```python
from build123d import *

# Parameters (mm, degrees)
SKETCH3_W           = 59
SKETCH3_H           = 36
SKETCH3_W_2         = 44
SKETCH3_H_2         = 21
BOSS_EXTRUDE1_DEPTH = 10
SKETCH3_2_W         = 59
SKETCH3_2_H         = 36
SKETCH3_2_W_2       = 44
SKETCH3_2_H_2       = 21
BOSS_EXTRUDE2_DEPTH = 5
SKETCH4_W           = 23.855112314
SKETCH4_H           = 12
BOSS_EXTRUDE3_DEPTH = 36.6
REVOLVE1_ANGLE      = 20
BOSS_EXTRUDE4_DEPTH = 10
BOSS_EXTRUDE5_REACH = 83.498
SKETCH9_W           = 12
SKETCH9_H           = 10.265164511
SKETCH3_4_W         = 59
SKETCH3_4_H         = 36
SKETCH3_4_W_2       = 44
SKETCH3_4_H_2       = 21
BOSS_EXTRUDE6_DEPTH = 7.65
BOSS_EXTRUDE7_START = 7.65
SKETCH3_5_W         = 59
SKETCH3_5_H         = 36
SKETCH3_5_W_2       = 44
SKETCH3_5_H_2       = 21
BOSS_EXTRUDE7_DEPTH = 25


with BuildPart() as part:
    # Sketch3 → Boss-Extrude1 (new body)
    with BuildSketch(Plane.XY):
        Rectangle(SKETCH3_W, SKETCH3_H)
        Rectangle(SKETCH3_W_2, SKETCH3_H_2, mode=Mode.SUBTRACT)
    extrude(amount=BOSS_EXTRUDE1_DEPTH)

    # Sketch3<2> → Boss-Extrude2 (add)
    # profile 1 of 2: a face of its own
    with BuildSketch(Plane.XY):
        Rectangle(SKETCH3_2_W, SKETCH3_2_H)
        Rectangle(SKETCH3_2_W_2, SKETCH3_2_H_2, mode=Mode.SUBTRACT)
    # profile 2 of 2: a face of its own
    with BuildSketch(Plane.XY):
        Rectangle(SKETCH3_2_W_2, SKETCH3_2_H_2)
    extrude(amount=-BOSS_EXTRUDE2_DEPTH)

    # Sketch4 → Boss-Extrude3 (add)
    with BuildSketch(Plane(origin=(0, 18, 0), x_dir=(1, 0, 0), z_dir=(0, 1, 0))):
        with Locations((0, -1)):
            Rectangle(SKETCH4_W, SKETCH4_H)
    extrude(amount=BOSS_EXTRUDE3_DEPTH)



with BuildPart() as body_2:
    # Sketch5 → Revolve1 (revolve, symmetric)
    with BuildSketch(Plane(origin=(0, 0, 0), x_dir=(0, 0, -1), z_dir=(1, 0, 0))) as revolve1_sk:
        with BuildLine():
            Line((6.375, 59.6), (-8.375, 59.6))
            ThreePointArc((-8.375, 59.6), (-2.924218778, 65.873958371), (4.625, 69.35))
            Line((4.625, 69.35), (6.375, 69.35))
            Line((6.375, 69.35), (6.375, 59.6))
        make_face()
    revolve(axis=Axis((0, -41.396267669, 52.68), (0, 1, 0)), revolution_arc=REVOLVE1_ANGLE / 2)
    revolve(revolve1_sk.sketch, axis=Axis((0, -41.396267669, 52.68), (0, -1, 0)), revolution_arc=REVOLVE1_ANGLE / 2)

    # Sketch7 → Boss-Extrude4 (add)
    with BuildSketch(Plane(origin=(-9.008810575, 0, 1.588496368), x_dir=(-0.17364817766693075, 0, -0.9848077530122081), z_dir=(0.9848077530122081, 0, -0.17364817766693075))):
        with BuildLine():
            Line((7.175327571, 59.6), (7.175327571, 66.343971629))
            Line((7.175327571, 66.343971629), (-0.614099568, 66.343971629))
            ThreePointArc((-0.614099568, 66.343971629), (-4.541815528, 63.433785776), (-7.574672429, 59.6))
            Line((-7.574672429, 59.6), (-7.574672429, 39.6))
            Line((-7.574672429, 39.6), (7.175327571, 39.6))
            Line((7.175327571, 39.6), (7.175327571, 59.6))
        make_face()
    extrude(amount=-BOSS_EXTRUDE4_DEPTH)


with BuildPart() as part_1:
    add(part.part)

    add(body_2.part)  # Boss-Extrude5 merges body 2
    # Boss-Extrude5: up to this plane
    boss_extrude5_end = Plane(origin=(-9.008810575, 0, 1.588496368), z_dir=(-0.9848077530122081, 0, 0.17364817766693075))
    # Sketch9 → Boss-Extrude5 (add, up to the surface)
    with BuildSketch(Plane(origin=(-11.927556157, 0, 0), x_dir=(0, 0, -1), z_dir=(1, 0, 0)), mode=Mode.PRIVATE) as boss_extrude5_sk1:
        with Locations((-1, 49.467417744)):
            Rectangle(SKETCH9_W, SKETCH9_H)
    boss_extrude5_tool1 = split(extrude(boss_extrude5_sk1.sketch, amount=BOSS_EXTRUDE5_REACH, mode=Mode.PRIVATE), bisect_by=boss_extrude5_end, keep=Keep.BOTH, mode=Mode.PRIVATE)
    add(boss_extrude5_tool1.solids().sort_by_distance((-11.927556, 49.467418, 1))[0])

    # Sketch3<4> → Boss-Extrude6 (add)
    # profile 1 of 2: a face of its own
    with BuildSketch(Plane.XY):
        Rectangle(SKETCH3_4_W, SKETCH3_4_H)
        Rectangle(SKETCH3_4_W_2, SKETCH3_4_H_2, mode=Mode.SUBTRACT)
    # profile 2 of 2: a face of its own
    with BuildSketch(Plane.XY):
        Rectangle(SKETCH3_4_W_2, SKETCH3_4_H_2)
    extrude(amount=BOSS_EXTRUDE6_DEPTH)

    # Sketch3<5> → Boss-Extrude7 (add)
    with BuildSketch(Plane.XY.offset(BOSS_EXTRUDE7_START)):
        Rectangle(SKETCH3_5_W, SKETCH3_5_H)
        Rectangle(SKETCH3_5_W_2, SKETCH3_5_H_2, mode=Mode.SUBTRACT)
    extrude(amount=BOSS_EXTRUDE7_DEPTH)


solid = part_1.part
```
Check sheet for the modelled part. Datum: model origin and axes. Units: mm. A direction names the side the tool comes from. Give positions to 0.01 mm unless a question says otherwise; leave off trailing zeros. Write each loop counter-clockwise with the first axis right and the second up, starting at its lowest first coordinate (ties: lowest second). Pieces come first, ordered by that corner, then holes.
Item 1: Scan lines: L1, parallel to Y at x = 5.5, z = 9.5; L2, parallel to X at y = -10, z = 16.5; L3, parallel to Y at x = 21, z = -0.5. Record each from-to range of solid material in increasing order.
Item 2: Cross-section at B-B (x = 14.5). Enter the section's corners in (y, z).
Item 3: Draft check along Y on faces 1 (the face through (0, -18, 14)), 2 (the face through (0, 69.35, -5)), 3 (the face through (-12.549, 49.74, 9.904)), 4 (the face through (0, 10.5, 20)). Enter one of: released by +Y, released by -Y, zero draft, split by the parting line, or undercut.
Item 4: Access from +Z, -Z, +X, -X, +Y, -Y to the whole of each face (thin tool, end or side, straight path). Record for faces 5 (the face through (-13.08, 63.48, 6.87)), 6 (the face through (11.928, 36, 1)), 7 (the face through (-22, 0, 20)), 8 (the face through (-18.804, 53.159, 3.623)), 9 (the face through (-29.5, 0, 14)).
Item 5: Cross-section at D-D (x = 0). Enter the section's corners in (y, z) (3 decimals), and give its area (3 significant figures).
Item 6: Cross-section at C-C (y = -2). Enter the section's corners in (x, z), and give its area (3 significant figures).
Item 7: Gauge pin test, flat ends, axial feed: pin 1 (6 mm diameter, centred on x = -13, z = 19, fed in from +Y); pin 2 (17 mm diameter, centred on x = 3, y = -0.5, fed in from +Z); pin 3 (1.5 mm diameter, centred on x = -17, y = 2.5, fed in from -Z); pin 4 (4 mm diameter, centred on x = 12.5, y = 59, fed in from +Z). Record the tip position at first contact, or that the pin passes through.
Item 8: Cross-section at A-A (z = 16). Enter the section's corners in (x, y).
Report:
1. L1: y = -18 to -10.5, 10.5 to 18
1. L2: x = -29.5 to -22, 22 to 29.5
1. L3: y = -18 to 18
2. outline: (-18, -5) - (18, -5) - (18, 32.65) - (10.5, 32.65) - (10.5, 7.65) - (-10.5, 7.65) - (-10.5, 32.65) - (-18, 32.65) - close
3. face 1: released by -Y
3. face 2: released by +Y
3. face 3: zero draft
3. face 4: undercut
4. face 5: +Z, +Y
4. face 6: +Z, -Z, +X, +Y
4. face 7: +Z
4. face 8: +Z, -X, +Y
4. face 9: +Z, -Z, -X, +Y, -Y
5. outline: (-18, -5) - (54.6, -5) - (54.6, 7) - (18, 7) - (18, 32.65) - (10.5, 32.65) - (10.5, 7.65) - (-10.5, 7.65) - (-10.5, 32.65) - (-18, 32.65) - close; (59.6, -6.375) - (69.35, -6.375) - (69.35, -4.625) arc R19.75 ccw to (59.6, 8.375) - close
5. area: 1,370 mm2
6. outline: (-29.5, -5) - (29.5, -5) - (29.5, 32.65) - (22, 32.65) - (22, 7.65) - (-22, 7.65) - (-22, 32.65) - (-29.5, 32.65) - close
6. area: 1,120 mm2
7. pin 1: stops at y = 18
7. pin 2: stops at z = 7.65
7. pin 3: stops at z = -5
7. pin 4: passes through
8. outline: (-29.5, -18) - (29.5, -18) - (29.5, 18) - (-29.5, 18) - close; hole (-22, -10.5) - (22, -10.5) - (22, 10.5) - (-22, 10.5) - close
